Part model, mm, in its own coordinate system. A direction names the side the tool comes from. Give positions to 0.01 mm unless a question says otherwise; leave off trailing zeros. Loops run counter-clockwise (first coordinate to the right, second up) from the corner with the lowest first, then second, coordinate; pieces in that order, holes last. Notation, with made-up numbers: M 56,42.25 L 74,42.25 A25 cw 74,56.25 Z; hole C 36.25,76 d7. An arc over 180 degrees is marked long. Answer in a Markdown table with one row per item.
from build123d import *

# Parameters (mm, degrees)
SKETCH1_W               = 60
SKETCH1_H               = 60
SKETCH1_R               = 21.25
BOSS_EXTRUDE1_DEPTH     = 12
SKETCH2_W               = 60
SKETCH2_H               = 60
SKETCH2_R               = 19.25
BOSS_EXTRUDE2_DEPTH     = 5
BOSS_EXTRUDE3_DEPTH     = 30
SKETCH4_W               = 15
SKETCH4_H               = 60
BOSS_EXTRUDE4_DEPTH     = 40
CUT_EXTRUDE1_DEPTH      = 212.381763641
CUT_EXTRUDE1_DEPTH_BACK = 212.381763641
SKETCH5_R               = 5.1
SKETCH6_R               = 2.75
CUT_EXTRUDE2_DEPTH      = 184.935450634
CHAMFER1_SIZE           = 15
FILLET1_R               = 1
FILLET2_R               = 1
FILLET3_R               = 2


with BuildPart() as part:
    # Sketch1 → Boss-Extrude1 (new body)
    with BuildSketch(Plane.XY):
        Rectangle(SKETCH1_W, SKETCH1_H)
        Circle(SKETCH1_R, mode=Mode.SUBTRACT)
    extrude(amount=BOSS_EXTRUDE1_DEPTH)

    # Sketch2 → Boss-Extrude2 (add)
    with BuildSketch(Plane.XY.offset(12)):
        Rectangle(SKETCH2_W, SKETCH2_H)
        Circle(SKETCH2_R, mode=Mode.SUBTRACT)
    extrude(amount=BOSS_EXTRUDE2_DEPTH)

    # Sketch3 → Boss-Extrude3 (add, symmetric)
    with BuildSketch(Plane(origin=(0, 0, 0), x_dir=(1, 0, 0), z_dir=(0, 1, 0))):
        Polygon((-30, 0), (-110, 0), (-110, 61.5), (-130, 61.5), (-130, -17), (-30, -17), align=None)
    extrude(amount=BOSS_EXTRUDE3_DEPTH, both=True)

    # Sketch4 → Boss-Extrude4 (add)
    with BuildSketch(Plane.ZY.offset(130)):
        with Locations((-54, 0)):
            Rectangle(SKETCH4_W, SKETCH4_H)
    extrude(amount=BOSS_EXTRUDE4_DEPTH)

    # Sketch5 → Cut-Extrude1 (cut, two sides: drawn at the far end of the back side and taken through both)
    with BuildSketch(Plane.ZY.offset(170).offset(-CUT_EXTRUDE1_DEPTH_BACK)):
        with Locations((-61.5, 0)):
            Circle(SKETCH5_R)
    extrude(amount=CUT_EXTRUDE1_DEPTH + CUT_EXTRUDE1_DEPTH_BACK, mode=Mode.SUBTRACT)

    # Sketch6 → Cut-Extrude2 (cut, through all)
    with BuildSketch(Plane.XY.offset(-46.5)):
        with Locations((-140, 17.5)):
            Circle(SKETCH6_R)
        with Locations(Location((-140, -17.5, 0), (0, 0, 180))):
            Circle(SKETCH6_R)
        with Locations((-160, -17.5)):
            Circle(SKETCH6_R)
        with Locations(Location((-160, 17.5, 0), (0, 0, 180))):
            Circle(SKETCH6_R)
    extrude(amount=-CUT_EXTRUDE2_DEPTH, mode=Mode.SUBTRACT)

    # Chamfer1
    chamfer1_edges = [part.edges().sort_by_distance(p)[0] for p in [
        (-110, 0, 0),
    ]]
    chamfer(chamfer1_edges, length=CHAMFER1_SIZE)

    # Fillet1
    fillet1_edges = [part.edges().sort_by_distance(p)[0] for p in [
        (-21.25, 0, 0),
    ]]
    fillet(fillet1_edges, radius=FILLET1_R)

    # Fillet2
    fillet2_edges = [part.edges().sort_by_distance(p)[0] for p in [
        (-19.25, 0, 17),
    ]]
    fillet(fillet2_edges, radius=FILLET2_R)

    # Fillet3
    fillet3_edges = [part.edges().sort_by_distance(p)[0] for p in [
        (-50, 30, 17),
        (-50, -30, 17),
        (30, 0, 17),
        (-130, 0, 17),
        (-130, -30, -14.75),
        (-130, 30, -14.75),
        (-130, 0, -46.5),
        (-150, -30, -46.5),
        (-150, 30, -46.5),
        (-170, -30, -54),
        (-170, 0, -46.5),
        (-170, 30, -54),
        (-32.5, 30, 0),
        (30, 0, 0),
        (30, -30, 8.5),
        (30, 30, 8.5),
        (-110, 30, -38.25),
        (-110, -30, -38.25),
        (-110, 0, -15),
        (-32.5, -30, 0),
        (-95, 0, 0),
        (-102.5, -30, -7.5),
        (-102.5, 30, -7.5),
    ]]
    fillet(fillet3_edges, radius=FILLET3_R)


solid = part.part
(1) Which spindle directions (+Z, -Z, +X, -X, +Y, -Y) get a long thin tool onto all of the face, cutting with end or side? Do faces 1 (the face through (-11, 16, 12)), 2 (the face through (-46, 0, 0)), 3 (the face through (-130, 0, -15)). Say none if no direction does.
Recorded:
| item | result |
|---|---|
| face 1 | -Z |
| face 2 | -Z, +X, +Y, -Y |
| face 3 | +Z, -X, +Y, -Y |
(2) Saw through at C-C (x = -140). Write the cut outline in (y, z), plus the area to 3 significant figures.
Recorded:
| item | result |
|---|---|
| outline | M -30,-61.5 L -20.25,-61.5 L -20.25,-46.5 L -28,-46.5 A2 ccw -30,-48.5 Z; M -14.75,-61.5 L -5.1,-61.5 A5.1 cw 5.1,-61.5 L 14.75,-61.5 L 14.75,-46.5 L -14.75,-46.5 Z; M 20.25,-61.5 L 30,-61.5 L 30,-48.5 A2 ccw 28,-46.5 L 20.25,-46.5 Z |
| area | 692 mm^2 |
(3) Saw through at D-D (z = -28.5). Write the cut outline in (x, y).
Recorded:
| item | result |
|---|---|
| outline | M -130,-28 A2 ccw -128,-30 L -112,-30 A2 ccw -110,-28 L -110,28 A2 ccw -112,30 L -128,30 A2 ccw -130,28 Z |
(4) Saw through at B-B (z = -52). Write the cut outline in (x, y), plus the area to 3 significant figures.
Recorded:
| item | result |
|---|---|
| outline | M -170,-28 A2 ccw -168,-30 L -112,-30 A2 ccw -110,-28 L -110,28 A2 ccw -112,30 L -168,30 A2 ccw -170,28 Z; hole C -160,-17.5 d5.5; hole C -160,17.5 d5.5; hole C -140,-17.5 d5.5; hole C -140,17.5 d5.5 |
| area | 3,500 mm^2 |
(5) Pull direction Y, two halves, no side cores. Call faces 4 (the face through (-162.62, 16.67, -53.9)), 5 (the face through (-102.83, 29.43, -6.98)), 6 (the face through (-139.6, -20.5, -61.5)), 7 (the face through (-99, -30, 2)): +Y half, -Y half, draft (parallel to the pull), parting line (faces both ways), or undercut.
Recorded:
| item | result |
|---|---|
| face 4 | undercut |
| face 5 | +Y half |
| face 6 | draft |
| face 7 | -Y half |
(6) Drill centre lines: line 1 along Y through (x, z) = (-160, -55); line 2 along Y through (x, z) = (0, 13); line 3 along Z through (x, y) = (-21.5, 26.5). Where is each one in solid material? Low to high.
Recorded:
| item | result |
|---|---|
| line 1 | y = -30 to -20.25, -14.75 to 14.75, 20.25 to 30 |
| line 2 | y = -30 to -19.25, 19.25 to 30 |
| line 3 | z = 0 to 17 |
(7) Saw through at A-A (y = 0). Write the cut outline in (x, z).
Recorded:
| item | result |
|---|---|
| outline | M -170,-56.4 L -110,-56.4 L -110,-15.83 A2 cw -109.41,-14.41 L -95.59,-0.59 A2 cw -94.17,0 L -22.25,0 A1 ccw -21.25,1 L -21.25,12 L -19.25,12 L -19.25,16 A1 ccw -20.25,17 L -128,17 A2 ccw -130,15 L -130,-44.5 A2 cw -132,-46.5 L -168,-46.5 A2 ccw -170,-48.5 Z; M 19.25,12 L 21.25,12 L 21.25,1 A1 ccw 22.25,0 L 28,0 A2 ccw 30,2 L 30,15 A2 ccw 28,17 L 20.25,17 A1 ccw 19.25,16 Z |
(8) Pin check, flat tips, straight feed: pin 1 Ø17 at (y, z) = (7, -10) entering from -X; pin 2 Ø7 at (x, y) = (-160, 17.5) entering from +Z; pin 3 Ø17 at (x, y) = (-53, 13.5) entering from -Z. Stop position of each tip, or through.
Recorded:
| item | result |
|---|---|
| pin 1 | stops at x = -130 |
| pin 2 | stops at z = -46.5 |
| pin 3 | stops at z = 0 |
